from build123d import *

# Parameters (mm, degrees)
SKETCH_1_R      = 2
SKETCH_1_R_2    = 8.5
EXTRUDE_1_DEPTH = 3
SKETCH_2_R      = 11
SKETCH_2_R_2    = 8.5
EXTRUDE_2_DEPTH = 1


with BuildPart() as part:
    # 草图1 → 凸台-拉伸1 (new body)
    with BuildSketch(Plane.XY):
        with BuildLine():
            Line((-12.519984026, -11.5), (12.519984026, -11.5))
            ThreePointArc((12.519984026, -11.5), (17, 0), (12.519984026, 11.5))
            Line((12.519984026, 11.5), (-12.519984026, 11.5))
            ThreePointArc((-12.519984026, 11.5), (-17, 0), (-12.519984026, -11.5))
        make_face()
        with Locations((-12, -7)):
            Circle(SKETCH_1_R, mode=Mode.SUBTRACT)
        with Locations((-12, 7)):
            Circle(SKETCH_1_R, mode=Mode.SUBTRACT)
        with Locations((12, 7)):
            Circle(SKETCH_1_R, mode=Mode.SUBTRACT)
        with Locations((12, -7)):
            Circle(SKETCH_1_R, mode=Mode.SUBTRACT)
        Circle(SKETCH_1_R_2, mode=Mode.SUBTRACT)
    extrude(amount=EXTRUDE_1_DEPTH)

    # 草图2 → 凸台-拉伸2 (add)
    with BuildSketch(Plane.XY.offset(3)):
        Circle(SKETCH_2_R)
        Circle(SKETCH_2_R_2, mode=Mode.SUBTRACT)
    extrude(amount=EXTRUDE_2_DEPTH)


solid = part.part
Geometry check sheet. Reference: the model listing, model coordinates, mm. A direction names the side the tool comes from. Round coordinates to 2 decimals unless told otherwise and drop trailing zeros. Loops run counter-clockwise (first coordinate to the right, second up) from the corner with the lowest first, then second, coordinate; pieces in that order, holes last. Notation, with made-up numbers: (-14, 70) -> (32, 70) arc R7 cw to (32, 76) -> close; hole circle Ø10 at (-35.75, 64.25). An arc over 180 degrees is marked (long way). Answer as a JSON object with one key per item and string values. Group by question number.
Item 1: Cross-section at D-D, the plane x = -12. Record the cut outline in (y, z), plus the area to 3 significant figures.
Item 2: Release check for a two-part mould opening along X. For faces 1 (the face through (0, -11.5, 1)), 2 (the face through (10, -7, 1)), 3 (the face through (-17, 0, 1)) record: pulls with the +X half, pulls with the -X half, needs draft (parallel to the pull), parting line crosses it, or undercut.
Item 3: Cross-section at C-C, the plane z = 1.7. Record the cut outline in (x, y), plus the area to 3 significant figures.
Item 4: Cross-section at A-A, the plane x = 0. Record the cut outline in (y, z), plus the area to 3 significant figures.
Item 5: Thickness scan on line 1 along Y through (x, z) = (12, 0.65); line 2 along Y through (x, z) = (0, 2.75); line 3 along X through (y, z) = (7.25, 1.65). Record the ranges inside material, lowest first.
Item 6: Cross-section at B-B, the plane y = 0. Record the cut outline in (x, z).
Item 7: Depth check by flat-ended pin: pin 1 Ø3.5 at (x, y) = (12, -7) entering from +Z; pin 2 Ø1.5 at (x, y) = (10.5, -6) entering from +Z. Enter the tip coordinate at first touch or a pass-through.
Item 8: Set-up check for faces 4 (the face through (4, 8, 0)), 5 (the face through (-2.38, -10.74, 3.49)): record each of +Z, -Z, +X, -X, +Y, -Y from which the full face is reachable in a straight line by a thin tool's end or side.
Determined:
{
 "1": {"outline": "(-11.5, 0) -> (-9, 0) -> (-9, 3) -> (-11.5, 3) -> close; (-5, 0) -> (5, 0) -> (5, 3) -> (-5, 3) -> close; (9, 0) -> (11.5, 0) -> (11.5, 3) -> (9, 3) -> close", "area": "45.0 mm²"},
 "2": {"face 1": "needs draft", "face 2": "undercut", "face 3": "pulls with the -X half"},
 "3": {"outline": "(-12.52, -11.5) -> (12.52, -11.5) arc R17 ccw to (12.52, 11.5) -> (-12.52, 11.5) arc R17 ccw to start; hole circle Ø4 at (-12, -7); hole circle Ø4 at (-12, 7); hole circle Ø17 at (0, 0); hole circle Ø4 at (12, -7); hole circle Ø4 at (12, 7)", "area": "440 mm²"},
 "4": {"outline": "(-11.5, 0) -> (-8.5, 0) -> (-8.5, 4) -> (-11, 4) -> (-11, 3) -> (-11.5, 3) -> close; (8.5, 0) -> (11.5, 0) -> (11.5, 3) -> (11, 3) -> (11, 4) -> (8.5, 4) -> close", "area": "23.0 mm²"},
 "5": {"line 1": "y = -11.5 to -9, -5 to 5, 9 to 11.5", "line 2": "y = -11.5 to -8.5, 8.5 to 11.5", "line 3": "x = -15.38 to -13.98, -10.02 to -4.44, 4.44 to 10.02, 13.98 to 15.38"},
 "6": {"outline": "(-17, 0) -> (-8.5, 0) -> (-8.5, 4) -> (-11, 4) -> (-11, 3) -> (-17, 3) -> close; (8.5, 0) -> (17, 0) -> (17, 3) -> (11, 3) -> (11, 4) -> (8.5, 4) -> close"},
 "7": {"pin 1": "passes through", "pin 2": "stops at z = 3"},
 "8": {"face 4": "-Z, +X, -X, +Y, -Y", "face 5": "+Z"}
}
